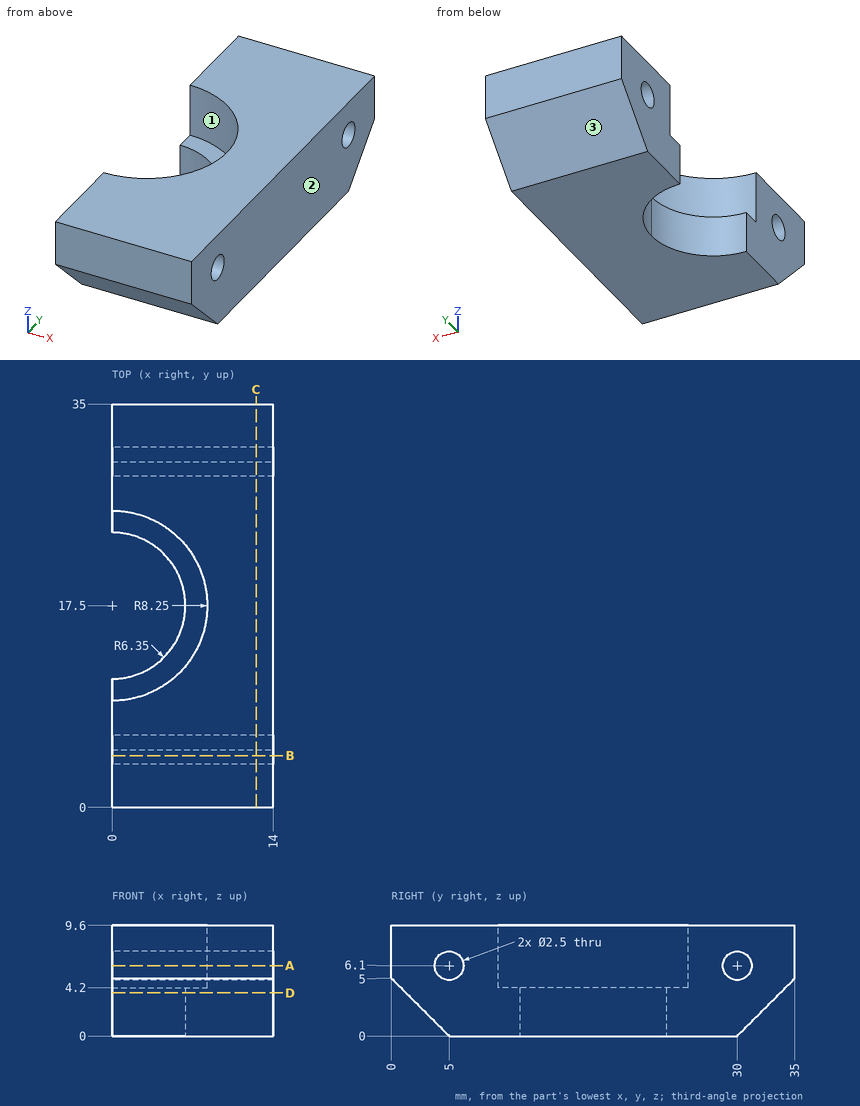
Print and shaded views of the part. All mm, measured from the part's lowest x, y and z. Coordinates: 2 decimals unless noted, no trailing zeros. Order: outer loops, then holes, each group sorted by start corner. A loop starts at its lowest first (then second) coordinate and runs counter-clockwise, first axis right, second up.
(1) Slice it at D-D, the plane z = 3.75. Write the cut outline in (x, y).
Check sheet entries:
outline: (0, 1.25) - (14, 1.25) - (14, 33.75) - (0, 33.75) - (0, 23.85) arc R6.35 cw to (0, 11.15) - close
(2) Slice it at C-C, the plane x = 12.5. Write the cut outline in (y, z), and give its area (3 significant figures).
Check sheet entries:
outline: (0, 5) - (5, 0) - (30, 0) - (35, 5) - (35, 9.6) - (0, 9.6) - close; hole circle Ø2.5 at (5, 6.1); hole circle Ø2.5 at (30, 6.1)
area: 301 mm2
(3) Pin check, flat tips, straight feed: pin 1 Ø1.5 at (y, z) = (18, 3.5) entering from -X; pin 2 Ø1 at (x, z) = (5.5, 1.5) entering from +Y; pin 3 Ø1.5 at (y, z) = (5, 6.1) entering from -X. Stop position of each tip, or through.
Check sheet entries:
pin 1: stops at x = 6.23
pin 2: stops at y = 32
pin 3: passes through
(4) Pull direction Y, two halves, no side cores. Call the marked faces 1, 2 and 3: pulls with the +Y half, pulls with the -Y half, needs draft (parallel to the pull), parting line crosses it, or undercut.
Check sheet entries:
face 1: undercut
face 2: needs draft
face 3: pulls with the +Y half
(5) Slice it at B-B, the plane y = 4.5. Write the cut outline in (x, z), and give its area (3 significant figures).
Check sheet entries:
outline: (0, 0.5) - (14, 0.5) - (14, 4.95) - (0, 4.95) - close; (0, 7.25) - (14, 7.25) - (14, 9.6) - (0, 9.6) - close
area: 95.3 mm2
(6) Probe L1, parallel to Y at x = 13.25, z = 6.25; L2, parallel to Z at x = 4.5, y = 11; L3, parallel to Z at x = 10.75, y = 6. List the from-to ranges inside material, lowest first.
Check sheet entries:
L1: y = 0 to 3.76, 6.24 to 28.76, 31.24 to 35
L2: z = 0 to 4.2
L3: z = 0 to 5.35, 6.85 to 9.6
(7) Slice it at A-A, the plane z = 6.1. Write the cut outline in (x, y), and give its area (3 significant figures).
Check sheet entries:
outline: (0, 0) - (14, 0) - (14, 3.75) - (0, 3.75) - close; (0, 6.25) - (14, 6.25) - (14, 28.75) - (0, 28.75) - (0, 25.75) arc R8.25 cw to (0, 9.25) - close; (0, 31.25) - (14, 31.25) - (14, 35) - (0, 35) - close
area: 313 mm2
